from build123d import *

# Parameters (mm, degrees)
PAD_DEPTH       = 250
SKETCH001_R     = 1.5
POCKET_DEPTH    = 8.15296
SKETCH002_R     = 3
POCKET001_DEPTH = 5


with BuildPart() as part:
    # Sketch → Pad (new body)
    with BuildSketch(Plane.XY):
        with BuildLine():
            Line((-5.5, 0), (5.5, 0))
            ThreePointArc((5.5, 0), (5.949397, 0.280814), (5.894005, 0.807831))
            Line((2.5, 5.15196), (5.894005, 0.807831))
            Line((5.768277, 7.230027), (2.5, 5.15196))
            ThreePointArc((5.768277, 7.230027), (5.980087, 7.791662), (5.5, 8.15196))
            Line((5.5, 8.15196), (-5.5, 8.15196))
            ThreePointArc((-5.5, 8.15196), (-5.980087, 7.791662), (-5.768277, 7.230027))
            Line((-5.768277, 7.230027), (-2.5, 5.15196))
            Line((-2.5, 5.15196), (-5.894005, 0.807831))
            ThreePointArc((-5.894005, 0.807831), (-5.949397, 0.280814), (-5.5, 0))
        make_face()
    extrude(amount=PAD_DEPTH)

    # Sketch001 (on Face2 of Pad) → Pocket (cut, through all)
    with BuildSketch(Plane(origin=(0, 8.15196, 0), x_dir=(-1, 0, 0), z_dir=(0, 1, 0))):
        with Locations((0, 10)):
            Circle(SKETCH001_R)
        with Locations((0, 35)):
            Circle(SKETCH001_R)
        with Locations((0, 60)):
            Circle(SKETCH001_R)
        with Locations((0, 85)):
            Circle(SKETCH001_R)
        with Locations((0, 110)):
            Circle(SKETCH001_R)
        with Locations((0, 135)):
            Circle(SKETCH001_R)
        with Locations((0, 160)):
            Circle(SKETCH001_R)
        with Locations((0, 185)):
            Circle(SKETCH001_R)
        with Locations((0, 210)):
            Circle(SKETCH001_R)
        with Locations((0, 235)):
            Circle(SKETCH001_R)
    extrude(amount=-POCKET_DEPTH, mode=Mode.SUBTRACT)

    # Sketch002 (on Face3 of Pocket) → Pocket001 (cut)
    with BuildSketch(Plane(origin=(0, 8.15196, 0), x_dir=(-1, 0, 0), z_dir=(0, 1, 0))):
        with Locations((0, 235)):
            Circle(SKETCH002_R)
        with Locations((0, 210)):
            Circle(SKETCH002_R)
        with Locations((0, 185)):
            Circle(SKETCH002_R)
        with Locations((0, 160)):
            Circle(SKETCH002_R)
        with Locations((0, 135)):
            Circle(SKETCH002_R)
        with Locations((0, 110)):
            Circle(SKETCH002_R)
        with Locations((0, 85)):
            Circle(SKETCH002_R)
        with Locations((0, 60)):
            Circle(SKETCH002_R)
        with Locations((0, 35)):
            Circle(SKETCH002_R)
        with Locations((0, 10)):
            Circle(SKETCH002_R)
    extrude(amount=-POCKET001_DEPTH, mode=Mode.SUBTRACT)


solid = part.part
Here's how the part is built. I have some questions about the finished solid (model axes, mm). A direction names the side the tool comes from. Coordinates: 2 decimals unless noted, no trailing zeros. Order: outer loops, then holes, each group sorted by start corner. A loop starts at its lowest first (then second) coordinate and runs counter-clockwise, first axis right, second up. Notation, with made-up numbers: (-39, 55.5) - (11, 55.5) arc R10 cw to (11, 62.5) - close; hole circle Ø1 at (17, 27.5). An arc over 180 degrees is marked (long way). Use CSV: the item, a comma, the result in double quotes. Start each with the question number.
1. I'm going to push flat-ended pins straight in: pin 1 (1.8 mm diameter, centred on x = 0, z = 210, fed in from +Y); pin 2 (3 mm diameter, centred on x = 1, z = 84, fed in from +Y); pin 3 (3 mm diameter, centred on y = 3.5, z = 79, fed in from -X). Where does each tip first touch, or does it pass through?
2. If we mould it in two halves opening along Z, with no side actions, what happens to faces 3 (the face through (0, 4, 0)), 4 (the face through (-1.3, 3.152, 33.7)), 5 (the face through (0, 0, 123))? For each: +Z half, -Z half, draft (parallel to the pull), parting line (faces both ways), or undercut.
3. Please list where these lines run through material, in increasing order: line 1 (Y direction, x = 4.25, z = 71.5); line 2 (X direction, y = 6.25, z = 60); line 3 (Y direction, x = -4.5, z = 159). Write a range as from..to.
4. Suppose I cut it at A-A on z = 173.5. List the corners of the cut face in (x, y) for me.
5. For faces 1 (the face through (-2.77, 5.69, 83.85)), 2 (the face through (0, 8.152, 123)), which set-ups out of +Z, -Z, +X, -X, +Y, -Y let a thin tool reach every point of the face, with its end or its side?
Output:
1,pin 1,"passes through"
1,pin 2,"stops at y = 3.15"
1,pin 3,"stops at x = -4.96"
2,face 3,"-Z half"
2,face 4,"undercut"
2,face 5,"draft"
3,line 1,"y = 0..2.91, 6.26..8.15"
3,line 2,"x = -4.23..-3, 3..4.23"
3,line 3,"y = 0..2.59, 6.42..8.15"
4,outline,"(-5.89, 0.81) arc R0.5 ccw to (-5.5, 0) - (5.5, 0) arc R0.5 ccw to (5.89, 0.81) - (2.5, 5.15) - (5.77, 7.23) arc R0.5 ccw to (5.5, 8.15) - (-5.5, 8.15) arc R0.5 ccw to (-5.77, 7.23) - (-2.5, 5.15) - close"
5,face 1,"+Y"
5,face 2,"+Z, -Z, +X, -X, +Y"
